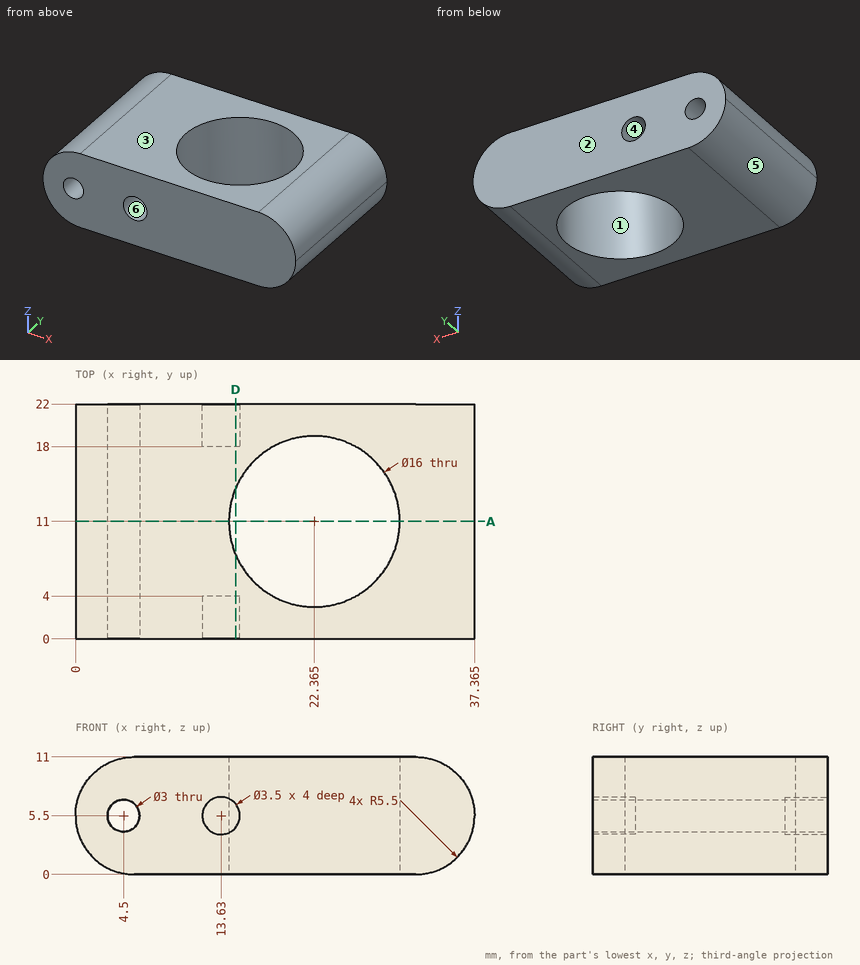
For this review, use the dimensioned drawing (mm, ordinates from the lowest corner) and the shaded views. A direction names the side the tool comes from. Give positions to 0.01 mm unless a question says otherwise; leave off trailing zeros. Write each loop counter-clockwise with the first axis right and the second up, starting at its lowest first coordinate (ties: lowest second). Pieces come first, ordered by that corner, then holes.
(1) Consider section A-A, the plane y = 11. Give the number of separate pieces and of enclosed holes in the cut face, and give its area (3 significant figures).
(2) Tool access review of the marked faces 4, 5 and 6: name each direction out of +Z, -Z, +X, -X, +Y, -Y from which nothing blocks a thin tool from reaching the whole face with its end or side.
(3) To check wall thickness, follow L1, parallel to X at y = 9, z = 5.5 (1 decimal); L2, parallel to Z at x = 13.63, y = 1.6; L3, parallel to X at y = 5, z = 5.25 (1 decimal). State the ranges of each line that lie inside material, in increasing order.
(4) Consider section D-D, the plane x = 15. Give the boundary of the cut face in (y, z).
(5) For P1, Ø1, axis at y = 12, z = 8, coming from the -X side; P2, Ø1.5, axis at y = 17, z = 8, coming from the -X side (1 decimal); P3, Ø2, axis at x = 13.63, z = 5.5, coming from the -Y side, all flat-tipped, find the tip position at first contact; note any pin that passes through.
(6) The part is to be moulded in two halves that separate along Y. For the marked faces 1, 2 and 3, say which applies: released by +Y, released by -Y, zero draft, split by the parting line, or undercut.
Returned:
1. separate pieces: 2
1. enclosed holes: 1
1. area: 202 mm2
2. face 4: +Y
2. face 5: -Z, -X, +Y, -Y
2. face 6: -Y
3. L1: x = 0 to 3, 6 to 14.6, 30.1 to 37.4
3. L2: z = 0 to 3.75, 7.25 to 11
3. L3: x = 0 to 3, 6 to 17.1, 27.7 to 37.4
4. outline: (0, 0) - (7.88, 0) - (7.88, 11) - (0, 11) - (0, 6.59) - (4, 6.59) - (4, 4.41) - (0, 4.41) - close; (14.12, 0) - (22, 0) - (22, 4.41) - (18, 4.41) - (18, 6.59) - (22, 6.59) - (22, 11) - (14.12, 11) - close
5. P1: stops at x = 0.38
5. P2: stops at x = 0.3
5. P3: stops at y = 4
6. face 1: undercut
6. face 2: released by +Y
6. face 3: zero draft
